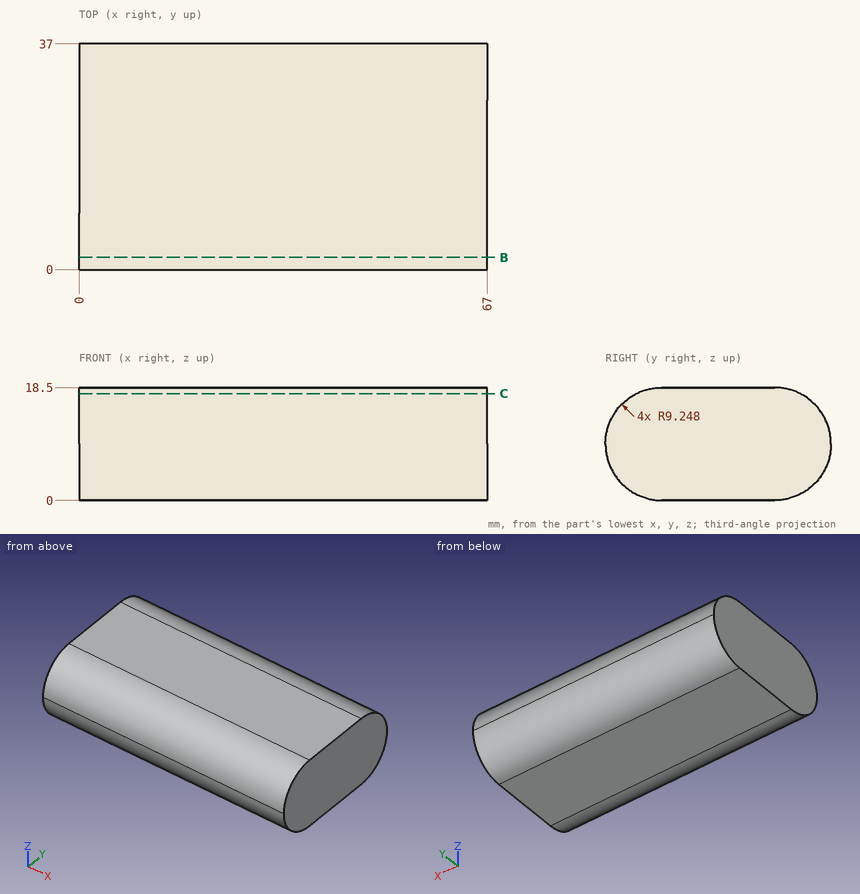
Geometry: see drawing. Coordinates: mm, zero at the bounding-box minimum. Give positions to 0.01 mm unless a question says otherwise; leave off trailing zeros. Loops run counter-clockwise (first coordinate to the right, second up) from the corner with the lowest first, then second, coordinate; pieces in that order, holes last. Notation, with made-up numbers: M 58,46 L 102,46 A10 cw 102,51 Z; hole C -40,25 d8. An arc over 180 degrees is marked long. Answer as CSV lines item,"result". Start each with the question number.
1. Section B-B on y = 2. Return loops of the section in (x, z), plus the area to 3 significant figures.
2. Pin query (flat end, axial travel): P1, Ø6, axis at x = 56.5, z = 12.5, coming from the -Y side; P2, Ø1, axis at x = 26.5, y = 4, coming from the -Z side. Return the tip coordinate at first contact, or that it passes through.
3. Line query: L1, parallel to Z at x = 26.5, y = 28; L2, parallel to Y at x = 36.5, z = 9.5; L3, parallel to Y at x = 61.5, z = 1.5. Output: solid intervals per line, ascending.
4. Section C-C on z = 17.5. Return loops of the section in (x, y) (1 decimal), plus the area to 3 significant figures.
Computed values:
1,outline,"M 0,3.5 L 67,3.5 L 67,15 L 0,15 Z"
1,area,"770 mm²"
2,P1,"stops at y = 0"
2,P2,"stops at z = 1.31"
3,L1,"z = 0 to 18.5"
3,L2,"y = 0 to 37"
3,L3,"y = 4.2 to 32.8"
4,outline,"M 0,5.1 L 67,5.1 L 67,31.9 L 0,31.9 Z"
4,area,"1,800 mm²"
